```python
from build123d import *

# Parameters (mm, degrees)
F3_DEPTH      = 5
F3_DEPTH_BACK = 5
F5_COUNT      = 6
F6_R          = 30
F7_DEPTH      = 20
F7_DEPTH_BACK = 20
F9_R          = 30
F10_DEPTH     = 25
F12_R         = 30
F13_DEPTH     = 25
F14_R         = 15
F15_DEPTH     = 25


with BuildPart() as f3:
    # F2 (on face) → F3 (new body, two sides)
    with BuildSketch(Plane(origin=(0, 0, 0), x_dir=(1, 0, 0), z_dir=(0, 0.5, -0.8660254038))) as f3_sk:
        with BuildLine():
            Line((0, -1.3531434218), (105.9060541663, -29.7305851092))
            ThreePointArc((105.9060541663, -29.7305851092), (110, 0), (105.9060541663, 29.7305851092))
            Line((105.9060541663, 29.7305851092), (-5.05, 0))
            Line((-5.05, 0), (0, 0))
            Line((0, 0), (0, -1.3531434218))
        make_face()
    extrude(amount=F3_DEPTH)
    extrude(f3_sk.sketch, amount=-F3_DEPTH_BACK)

    # F5: F3 ×6 about axis
    f5_axis = Axis((0, 0, 14.0805), (0, 0, 1))


with BuildPart() as f3_1:
    add(f3.part)
    for i in range(1, F5_COUNT):
        add(f3.part.rotate(f5_axis, i * 360 / F5_COUNT))

    # F6 (on Top) → F7 (join, two sides)
    with BuildSketch(Plane.XY) as f7_sk:
        Circle(F6_R)
    extrude(amount=F7_DEPTH)
    extrude(f7_sk.sketch, amount=-F7_DEPTH_BACK)

    # F9 (on plane+point) → F10 (cut)
    with BuildSketch(Plane.XY.offset(8.9574447446)):
        Circle(F9_R)
    extrude(amount=F10_DEPTH, mode=Mode.SUBTRACT)

    # F12 (on plane+point) → F13 (cut)
    with BuildSketch(Plane.XY.offset(-8.9574447446)):
        Circle(F12_R)
    extrude(amount=-F13_DEPTH, mode=Mode.SUBTRACT)

    # F14 (on face) → F15 (cut)
    with BuildSketch(Plane(origin=(0, 0, -8.9574447446), x_dir=(1, 0, 0), z_dir=(0, 0, -1))):
        Circle(F14_R)
    extrude(amount=-F15_DEPTH, mode=Mode.SUBTRACT)


solid = f3_1.part
```
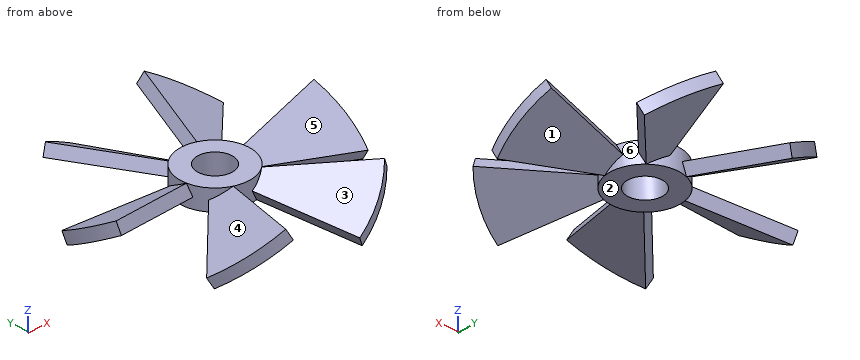
The listing builds one solid part. Answer for the finished solid, in the listing's coordinates (mm). Face numbers are marked on the shaded views. A direction names the side the tool comes from. Give positions to 0.01 mm unless a question says otherwise; leave off trailing zeros. Order: outer loops, then holes, each group sorted by start corner. A loop starts at its lowest first (then second) coordinate and runs counter-clockwise, first axis right, second up.
1) Find section A-A on x = 0. Write down the section's boundary in (y, z).
Reported:
outline: (-30, -8.96) - (-15, -8.96) - (-15, 8.96) - (-30, 8.96) - close; (15, -8.96) - (30, -8.96) - (30, 8.96) - (15, 8.96) - close
2) Given P1, Ø6, axis at y = 18, z = 2, coming from the +X side; P2, Ø18, axis at x = -1.5, y = 7.5, coming from the -Z side; P3, Ø2, axis at y = 31, z = 5.5, coming from the -X side, each flat-ended and moving along its own axis, determine where each tip first touches the part or whether it passes through.
Reported:
P1: stops at x = 109.02
P2: stops at z = -8.96
P3: stops at x = -32.55
3) Find section C-C on z = -14. Give the number of separate pieces and of enclosed holes in the cut face, then the cut area to 3 significant figures.
Reported:
separate pieces: 6
enclosed holes: 0
area: 1,490 mm2
4) Find section B-B on y = 41.5. Write down the section's boundary in (x, z).
Reported:
outline: (-43.68, 4.09) - (-13.99, -10.76) - (-8.9, -1.76) - (-37.02, 12.3) - close; (8.9, 1.76) - (37.02, -12.3) - (43.68, -4.09) - (13.99, 10.76) - close
5) Consider line 1 along X through (y, z) = (0, 3); line 2 along Y through (x, z) = (0, 0); line 3 along X through (y, z) = (-68.5, -0.5). Determine where each line is inside the solid, lowest interval first.
Reported:
line 1: x = -109.99 to -15, 15 to 109.99
line 2: y = -30 to -15, 15 to 30
line 3: x = -52.1 to -29, 27 to 50.1
6) Determine the mould class of the marked faces 4, 5 and 6 for opening direction X: pulls with the +X half, pulls with the -X half, needs draft (parallel to the pull), parting line crosses it, or undercut.
Reported:
face 4: pulls with the -X half
face 5: needs draft
face 6: undercut
7) For the marked faces 1, 2 and 3, determine the directions among +Z, -Z, +X, -X, +Y, -Y from which every point of the face is accessible in a straight line to the end or side of a thin tool.
Reported:
face 1: -Z, +X
face 2: -Z
face 3: +Z, -Y
